Source: CAD feature listing. Evaluate the final solid. Frame: model axes, mm. A direction names the side the tool comes from. Give positions to 0.01 mm unless a question says otherwise; leave off trailing zeros. Loops run counter-clockwise (first coordinate to the right, second up) from the corner with the lowest first, then second, coordinate; pieces in that order, holes last. Notation, with made-up numbers: M 19,42.25 L 26,42.25 A21 cw 26,60.25 Z; hole C -2,-4.5 d5. An arc over 180 degrees is marked long. Answer in a Markdown table with one row per item.
```python
from build123d import *

# Parameters (mm, degrees)
SKETCH_1_R          = 10
SKETCH_1_R_2        = 4.99999999999999
SKETCH_1_W          = 121.3397459621556
SKETCH_1_H          = 9.99999999999998
EXTRUDE_1_DEPTH     = 6
FILLET_1_R          = 4
SKETCH_3_R          = 5
CUT_EXTRUDE_1_DEPTH = 6
SKETCH_4_R          = 2.4999999999999982
EXTRUDE_2_DEPTH     = 5


with BuildPart() as part:
    # 草图1 → 凸台-拉伸1 (new body)
    with BuildSketch(Plane(origin=(0, 0, 0), x_dir=(1, 0, 0), z_dir=(0, 1, 0))):
        Circle(SKETCH_1_R)
        with Locations((130, 0)):
            Circle(SKETCH_1_R_2)
        with Locations((69.3301270189222, 0)):
            Rectangle(SKETCH_1_W, SKETCH_1_H)
    extrude(amount=EXTRUDE_1_DEPTH)

    # 草图2 → 旋转6 (revolve)
    with BuildSketch(Plane(origin=(0, 3, 0), x_dir=(1, 0, 0), z_dir=(0, 1, 0)), mode=Mode.PRIVATE) as revolve_6_sk:
        with BuildLine():
            ThreePointArc((130, -4.999999999999993), (133.53553390593277, -3.5355339059327036), (135, 8.296e-14))
            Line((135, 0), (130, 0))
            Line((130, 0), (122, 0))
            ThreePointArc((121.99999999999999, 9.8e-16), (122.45149074362405, -2.6495297708096603), (123.75500200160165, -5.0000000000000915))
            Line((123.7550020016017, -4.99999999999999), (130, -4.99999999999999))
        make_face()
        with BuildLine():
            ThreePointArc((123.75500200160165, -5.0000000000000915), (132.64952977080966, -7.548509256375958), (138, -1.96e-15))
            Line((138, 0), (135, 0))
            ThreePointArc((135, 8.296e-14), (133.53553390593277, -3.5355339059327036), (130, -4.999999999999993))
            Line((130, -4.99999999999999), (123.7550020016017, -4.99999999999999))
        make_face()
        with BuildLine():
            ThreePointArc((130, -4.999999999999993), (133.53553390593277, -3.5355339059327036), (135, 8.296e-14))
            Line((135, 0), (130, 0))
            Line((130, 0), (122, 0))
            ThreePointArc((121.99999999999999, 9.8e-16), (122.45149074362405, -2.6495297708096603), (123.75500200160165, -5.0000000000000915))
            Line((123.7550020016017, -4.99999999999999), (130, -4.99999999999999))
        make_face()
    revolve(revolve_6_sk.sketch.rotate(Axis((130, 3, 0), (1, 0, 0)), 180), axis=Axis((130, 3, 0), (1, 0, 0)))

    # 圆角1
    fillet_1_edges = [part.edges().sort_by_distance(p)[0] for p in [
        (123.7550020016015, 3.0000000000000013, 4.99999999999999),
        (122.58380151290432, 6, 7.053e-14),
        (123.94998914244879, 4.548343832458719, -4.99999999999999),
        (122.58380151290432, 0, 6.78e-14),
        (8.66025403784439, 3, -4.99999999999999),
        (8.66025403784439, 3, 4.99999999999999),
    ]]
    fillet(fillet_1_edges, radius=FILLET_1_R)

    # 草图3 → 切除-拉伸1 (cut)
    with BuildSketch(Plane.XZ):
        with Locations(Location((0, 0, 0), (0, 0, 270))):
            Circle(SKETCH_3_R)
    extrude(amount=-CUT_EXTRUDE_1_DEPTH, mode=Mode.SUBTRACT)

    # 草图4 → 凸台-拉伸2 (add)
    with BuildSketch(Plane.XZ):
        with Locations(Location((20, 0, 0), (0, 0, 90))):
            Circle(SKETCH_4_R)
    extrude(amount=EXTRUDE_2_DEPTH)


solid = part.part
```
1) Pin query (flat end, axial travel): pin 1 Ø8 at (x, z) = (0, 0) entering from -Y; pin 2 Ø3 at (x, z) = (60, -3.5) entering from +Y; pin 3 Ø8 at (x, y) = (82.5, 2.5) entering from +Z; pin 4 Ø2 at (x, z) = (49.5, -4.5) entering from -Y. Return the tip coordinate at first contact, or that it passes through.
Reply:
| item | result |
|---|---|
| pin 1 | passes through |
| pin 2 | stops at y = 6 |
| pin 3 | stops at z = 5 |
| pin 4 | stops at y = 0 |
2) Section A-A, the plane x = 0. Return loops of the section in (y, z).
Reply:
| item | result |
|---|---|
| outline | M 0,-10 L 6,-10 L 6,-5 L 0,-5 Z; M 0,5 L 6,5 L 6,10 L 0,10 Z |
3) Section D-D, the plane y = 9.5. Return loops of the section in (x, z).
Reply:
| item | result |
|---|---|
| outline | C 130,0 d9.33 |
4) Pull-direction query (X, two-part tool) for faces 1 (the flat face through (55, 6, 0)), 2 (the cylindrical face through (9.056, 3.042, -5.364)); classes: released by +X, released by -X, zero draft, split by the parting line, or undercut.
Reply:
| item | result |
|---|---|
| face 1 | zero draft |
| face 2 | undercut |
5) Section B-B, the plane x = 20. Return loops of the section in (y, z), then the cut area to 3 significant figures.
Reply:
| item | result |
|---|---|
| outline | M -5,-2.5 L 0,-2.5 L 0,-5 L 6,-5 L 6,5 L 0,5 L 0,2.5 L -5,2.5 Z |
| area | 85.0 mm² |
6) Material intervals for L1, parallel to Z at x = 108, y = 3.25; L2, parallel to Y at x = 85, z = -3.75; L3, parallel to X at y = -3.5, z = -0.5, sorted ascending.
Reply:
| item | result |
|---|---|
| L1 | z = -5 to 5 |
| L2 | y = 0 to 6 |
| L3 | x = 17.55 to 22.45, 125.36 to 134.64 |
7) Section C-C, the plane y = -3.5. Return loops of the section in (x, z), then the cut area to 3 significant figures.
Reply:
| item | result |
|---|---|
| outline | C 20,0 d5; C 130,0 d9.33 |
| area | 88.0 mm² |
8) Set-up query: faces 3 (the flat face through (66, 3, -5)), 4 (the cylindrical face through (17.89, -2.46, 1.34)), 5 (the flat face through (66, 3, 5)). Return all of +Z, -Z, +X, -X, +Y, -Y with unobstructed straight access to the full face (end or side cutting, diameter ignored); none if empty.
Reply:
| item | result |
|---|---|
| face 3 | -Z, +Y, -Y |
| face 4 | -Y |
| face 5 | +Z, +Y, -Y |
